Check sheet for the modelled part. Datum: model origin and axes. Units: mm. A direction names the side the tool comes from. Coordinates: 2 decimals unless noted, no trailing zeros. Order: outer loops, then holes, each group sorted by start corner. A loop starts at its lowest first (then second) coordinate and runs counter-clockwise, first axis right, second up.
from build123d import *

# Parameters (mm, degrees)
SKETCH1_R             = 2.425
BOSS_EXTRUDE1_DEPTH   = 7.5
BOSS_EXTRUDE1_2_DEPTH = 7.5
SKETCH2_W             = 60
SKETCH2_H             = 60
BOSS_EXTRUDE2_DEPTH   = 2.5


with BuildPart() as part:
    # Sketch1 → Boss-Extrude1 (new body)
    with BuildSketch(Plane(origin=(0, 0, 0), x_dir=(1, 0, 0), z_dir=(0, 1, 0))):
        with Locations(Location((-7.5, 0, 0), (0, 0, 270))):
            Circle(SKETCH1_R)
    extrude(amount=BOSS_EXTRUDE1_DEPTH)



with BuildPart() as body_2:
    # Sketch1 → Boss-Extrude1 2 (new body)
    with BuildSketch(Plane(origin=(0, 0, 0), x_dir=(1, 0, 0), z_dir=(0, 1, 0))):
        with Locations(Location((7.5, 0, 0), (0, 0, 270))):
            Circle(SKETCH1_R)
    extrude(amount=BOSS_EXTRUDE1_2_DEPTH)


with BuildPart() as part_1:
    add(part.part)

    add(body_2.part)  # Boss-Extrude2 merges body 2
    # Sketch2 → Boss-Extrude2 (add)
    with BuildSketch(Plane(origin=(0, 0, 0), x_dir=(1, 0, 0), z_dir=(0, 1, 0))):
        Rectangle(SKETCH2_W, SKETCH2_H)
    extrude(amount=-BOSS_EXTRUDE2_DEPTH)


solid = part_1.part
(1) Tool access check on faces 5 (the cylindrical face through (-9.65, 3.7, 1.12)), 6 (the flat face through (-7, 7.5, 0)). Record the directions out of +Z, -Z, +X, -X, +Y, -Y that give a thin tool (end or side, any length) a straight path to the whole face; none if there is none.
Filled in:
face 5: +Y
face 6: +Z, -Z, +X, -X, +Y
(2) Cross-section at B-B (y = 4.5). Enter the section's corners in (x, z) (3 decimals).
Filled in:
outline: circle Ø4.85 at (-7.5, 0); circle Ø4.85 at (7.5, 0)
(3) Cross-section at C-C (z = 0). Enter the section's corners in (x, y) (3 decimals), and give its area (3 significant figures).
Filled in:
outline: (-30, -2.5) - (30, -2.5) - (30, 0) - (9.925, 0) - (9.925, 7.5) - (5.075, 7.5) - (5.075, 0) - (-5.075, 0) - (-5.075, 7.5) - (-9.925, 7.5) - (-9.925, 0) - (-30, 0) - close
area: 223 mm2
(4) Go/stop test with a flat-tipped pin: P1, Ø12, axis at x = -20, z = 5, coming from the +Y side. Record where the tip stops, or that it passes through.
Filled in:
P1: stops at y = 0
(5) Thickness scan on probe 1 along Y at (x, z) = (7.5, 26); probe 2 along X at (y, z) = (7, -2); probe 3 along Z at (x, y) = (-8, 6.5). Record the ranges inside material, lowest first.
Filled in:
probe 1: y = -2.5 to 0
probe 2: x = -8.87 to -6.13, 6.13 to 8.87
probe 3: z = -2.37 to 2.37
(6) Cross-section at D-D (x = -2.5). Enter the section's corners in (y, z), and give its area (3 significant figures).
Filled in:
outline: (-2.5, -30) - (0, -30) - (0, 30) - (-2.5, 30) - close
area: 150 mm2
(7) Release check for a two-part mould opening along X. For faces 1 (the cylindrical face through (9.904, 3.698, -0.316)), 2 (the flat face through (0, -1, -30)), 3 (the flat face through (30, -1, 0)), 4 (the flat face through (-30, -1, 0)) record: +X half, -X half, draft (parallel to the pull), parting line (faces both ways), or undercut.
Filled in:
face 1: undercut
face 2: draft
face 3: +X half
face 4: -X half
(8) Cross-section at A-A (x = 7.5). Enter the section's corners in (y, z) (3 decimals), and give its area (3 significant figures).
Filled in:
outline: (-2.5, -30) - (0, -30) - (0, -2.425) - (7.5, -2.425) - (7.5, 2.425) - (0, 2.425) - (0, 30) - (-2.5, 30) - close
area: 186 mm2
